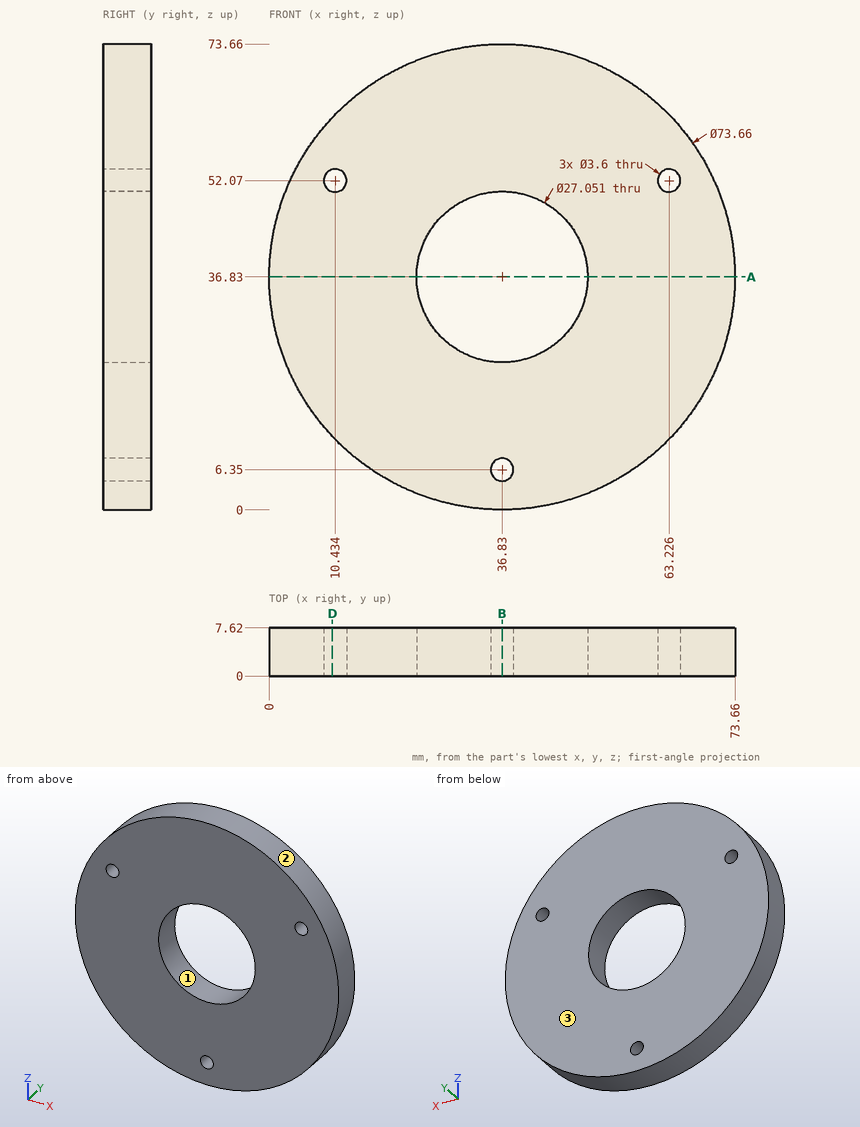
Can you work these out from the drawing? Everything is in mm from the part's minimum corner. Coordinates: 2 decimals unless noted, no trailing zeros. Write each loop counter-clockwise with the first axis right and the second up, starting at its lowest first coordinate (ties: lowest second). Pieces come first, ordered by that corner, then holes. Notation, with made-up numbers: (-16, -25) -> (36, -25) arc R27 cw to (36, 11) -> close; hole circle Ø1 at (49.25, -40). An arc over 180 degrees is marked (long way). Return JSON: item names as keys, results as strings.
(1) Imagine slicing it at A-A, the plane z = 36.83. Please give me the cut outline in (x, y) (1 decimal), then the cut area to 3 significant figures.
Numbers:
{"outline": "(0, 0) -> (23.3, 0) -> (23.3, 7.6) -> (0, 7.6) -> close; (50.4, 0) -> (73.7, 0) -> (73.7, 7.6) -> (50.4, 7.6) -> close", "area": "355 mm2"}
(2) I'm going to push flat-ended pins straight in: pin 1 (1 mm diameter, centred on y = 6, z = 30.5, fed in from -X) (1 decimal); pin 2 (2 mm diameter, centred on x = 7.5, y = 4, fed in from +Z) (1 decimal); pin 3 (3 mm diameter, centred on x = 52.5, y = 4.5, fed in from +Z) (1 decimal). Where does each tip first touch, or does it pass through?
Numbers:
{"pin 1": "stops at x = 0.5", "pin 2": "stops at z = 60.4", "pin 3": "stops at z = 70.8"}
(3) Imagine slicing it at D-D, the plane x = 10. Please give me the cut outline in (y, z).
Numbers:
{"outline": "(0, 11.6) -> (7.62, 11.6) -> (7.62, 50.32) -> (0, 50.32) -> close; (0, 53.82) -> (7.62, 53.82) -> (7.62, 62.06) -> (0, 62.06) -> close"}
(4) I need wall thicknesses on L1, parallel to X at y = 6, z = 36.83 (1 decimal); L2, parallel to X at y = 4.75, z = 52.07 (1 decimal); L3, parallel to Z at x = 38, y = 3.5 (1 decimal). Which ranges of each line are inside material? Lowest first, please.
Numbers:
{"L1": "x = 0 to 23.3, 50.4 to 73.7", "L2": "x = 3.3 to 8.6, 12.2 to 61.4, 65 to 70.4", "L3": "z = 0 to 5, 7.7 to 23.4, 50.3 to 73.6"}
(5) We'd pull the mould along Z, two halves only. Please class the marked faces 1, 2 and 3: +Z half, -Z half, draft (parallel to the pull), parting line (faces both ways), or undercut.
Numbers:
{"face 1": "undercut", "face 2": "parting line", "face 3": "draft"}
(6) Imagine slicing it at B-B, the plane x = 36.83. Count the separate pieces of the cut face and the enclosed holes in it, then the cut area to 3 significant figures.
Numbers:
{"separate pieces": "3", "enclosed holes": "0", "area": "328 mm2"}
